Study the drawing (mm; zero at the part's minimum x, y, z) and answer. A direction names the side the tool comes from. Give positions to 0.01 mm unless a question says otherwise; leave off trailing zeros. Write each loop counter-clockwise with the first axis right and the second up, starting at its lowest first coordinate (ties: lowest second). Pieces come first, ordered by that corner, then holes. Notation, with made-up numbers: (8, -17.75) - (27, -17.75) arc R22 ccw to (27, -3.75) - close; hole circle Ø11 at (-3.75, 36). An arc over 180 degrees is marked (long way). Return JSON: item names as keys, results as strings.
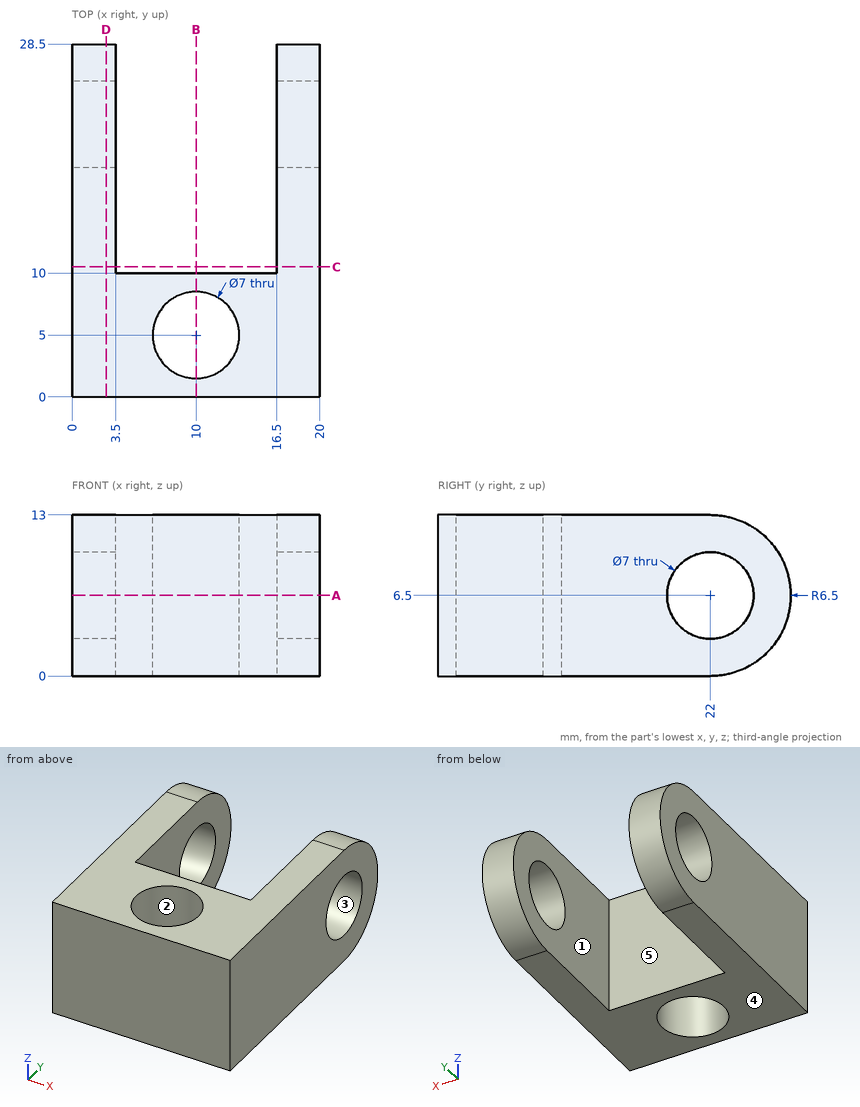
Item 1: The mould has two halves that part along Z. Classify the marked faces 3, 4 and 5: +Z half, -Z half, draft (parallel to the pull), parting line (faces both ways), or undercut.
Answer below:
{"face 3": "undercut", "face 4": "-Z half", "face 5": "draft"}
Item 2: A cutting plane is placed at B-B on x = 10. Determine the outline of the cut face in (y, z).
Answer below:
{"outline": "(0, 0) - (1.5, 0) - (1.5, 13) - (0, 13) - close; (8.5, 0) - (10, 0) - (10, 13) - (8.5, 13) - close"}
Item 3: Consider L1, parallel to Y at x = 19.1, z = 6.5; L2, parallel to X at y = 27.25, z = 5.5; L3, parallel to Z at x = 17.6, y = 22. Determine where each line is inside the solid, lowest interval first.
Answer below:
{"L1": "y = 0 to 18.5, 25.5 to 28.5", "L2": "x = 0 to 3.5, 16.5 to 20", "L3": "z = 0 to 3, 10 to 13"}
Item 4: A cutting plane is placed at C-C on y = 10.5. Determine the outline of the cut face in (x, z), then the cut area to 3 significant figures.
Answer below:
{"outline": "(0, 0) - (3.5, 0) - (3.5, 13) - (0, 13) - close; (16.5, 0) - (20, 0) - (20, 13) - (16.5, 13) - close", "area": "91.0 mm²"}
Item 5: A cutting plane is placed at D-D on x = 2.75. Determine the outline of the cut face in (y, z), then the cut area to 3 significant figures.
Answer below:
{"outline": "(0, 0) - (22, 0) arc R6.5 ccw to (22, 13) - (0, 13) - close; hole circle Ø7 at (22, 6.5)", "area": "314 mm²"}
Item 6: A flat-ended cylindrical pin translates along its axis: P1, Ø4, axis at x = 10.5, z = 8, coming from the +Y side. Find the tip coordinate at first contact, or state that the pin passes through.
Answer below:
{"P1": "stops at y = 10"}
Item 7: A cutting plane is placed at A-A on z = 6.5. Determine the outline of the cut face in (x, y), then the cut area to 3 significant figures.
Answer below:
{"outline": "(0, 0) - (20, 0) - (20, 18.5) - (16.5, 18.5) - (16.5, 10) - (3.5, 10) - (3.5, 18.5) - (0, 18.5) - close; (0, 25.5) - (3.5, 25.5) - (3.5, 28.5) - (0, 28.5) - close; (16.5, 25.5) - (20, 25.5) - (20, 28.5) - (16.5, 28.5) - close; hole circle Ø7 at (10, 5)", "area": "242 mm²"}
Item 8: For the marked faces 1 and 2, determine the directions among +Z, -Z, +X, -X, +Y, -Y from which every point of the face is accessible in a straight line to the end or side of a thin tool.
Answer below:
{"face 1": "+Z, -Z, +Y", "face 2": "+Z, -Z"}
